Build history of the part. All positions in model axes, mm. A direction names the side the tool comes from. Round coordinates to 2 decimals unless told otherwise and drop trailing zeros. Order: outer loops, then holes, each group sorted by start corner. A loop starts at its lowest first (then second) coordinate and runs counter-clockwise, first axis right, second up. Notation, with made-up numbers: (29, 74.5) -> (64, 74.5) arc R30 cw to (64, 105.5) -> close; hole circle Ø10 at (84, 53.5). An arc over 180 degrees is marked (long way). Answer as a JSON object with one key per item and string values.
from build123d import *

# Parameters (mm, degrees)
BOSS_EXTRUDE1_DEPTH   = 3.175
BOSS_EXTRUDE2_DEPTH   = 3.175
F_4_CLEARANCE_HOLE1_D = 2.9464


with BuildPart() as part:
    # Sketch1 → Boss-Extrude1 (new body)
    with BuildSketch(Plane(origin=(0, 0, -14.15699402), x_dir=(-1, 0, 0), z_dir=(0, 0, -1))):
        with BuildLine():
            Line((-49.172312317, -34.502108483), (-53.141062317, -27.628031841))
            ThreePointArc((-53.141062317, -27.628031841), (-55.063803638, -24.012221257), (-56.72992661, -20.271224785))
            ThreePointArc((-56.72992661, -20.271224785), (-54.976138042, -16.13776671), (-50.842679967, -17.891555277))
            ThreePointArc((-50.842679967, -17.891555277), (-49.356678398, -21.228119699), (-47.641801003, -24.453031841))
            Line((-47.641801003, -24.453031841), (-43.673051003, -31.327108483))
            ThreePointArc((-43.673051003, -31.327108483), (-16.68272836, -52.037511462), (17.046778195, -47.596937682))
            Line((17.046778195, -47.596937682), (23.920854837, -43.628187682))
            Line((23.920854837, -43.628187682), (30.79493148, -39.659437682))
            ThreePointArc((30.79493148, -39.659437682), (51.505334458, -12.669115038), (47.064760678, 21.060391517))
            Line((47.064760678, 21.060391517), (43.096010678, 27.934468159))
            ThreePointArc((43.096010678, 27.934468159), (41.160593535, 31.032051618), (39.01404477, 33.987248938))
            ThreePointArc((39.01404477, 33.987248938), (39.561948355, 38.44382292), (44.018522337, 37.895919335))
            ThreePointArc((44.018522337, 37.895919335), (46.425258832, 34.58251628), (48.595271992, 31.109468159))
            Line((48.595271992, 31.109468159), (52.564021992, 24.235391517))
            ThreePointArc((52.564021992, 24.235391517), (57.638963455, -14.312615975), (33.96993148, -45.158698996))
            Line((33.96993148, -45.158698996), (27.095854837, -49.127448996))
            Line((27.095854837, -49.127448996), (20.221778195, -53.096198996))
            ThreePointArc((20.221778195, -53.096198996), (-18.326229296, -58.171140459), (-49.172312317, -34.502108483))
        make_face()
    extrude(amount=BOSS_EXTRUDE1_DEPTH)

    # Sketch6 → Boss-Extrude2 (add)
    with BuildSketch(Plane.XY.offset(-14.15699402)):
        Polygon((78.577241059, -56.126600757), (56.126600757, -78.577241059), (27.345741417, -49.796381719), (49.796381719, -27.345741417), align=None)
        with BuildLine():
            Line((62.053569797, -46.248319024), (64.873370219, -49.068119446))
            ThreePointArc((64.873370219, -49.068119446), (64.873370219, -64.873370219), (49.068119446, -64.873370219))
            Line((49.068119446, -64.873370219), (46.248319024, -62.053569797))
            ThreePointArc((46.248319024, -62.053569797), (46.248319024, -46.248319024), (62.053569797, -46.248319024))
        make_face(mode=Mode.SUBTRACT)
        with BuildLine():
            Line((55.946995634, -74.266718121), (53.127195212, -71.446917699))
            ThreePointArc((53.127195212, -71.446917699), (53.127195212, -69.399419304), (55.174693608, -69.399419304))
            Line((55.174693608, -69.399419304), (57.99449403, -72.219219726))
            ThreePointArc((57.99449403, -72.219219726), (57.99449403, -74.266718121), (55.946995634, -74.266718121))
        make_face(mode=Mode.SUBTRACT)
        with BuildLine():
            Line((38.902469516, -53.127195212), (41.722269938, -55.946995634))
            ThreePointArc((41.722269938, -55.946995634), (41.722269938, -57.99449403), (39.674771543, -57.99449403))
            Line((39.674771543, -57.99449403), (36.854971121, -55.174693608))
            ThreePointArc((36.854971121, -55.174693608), (36.854971121, -53.127195212), (38.902469516, -53.127195212))
        make_face(mode=Mode.SUBTRACT)
        with BuildLine():
            Line((55.174693608, -36.854971121), (57.99449403, -39.674771543))
            ThreePointArc((57.99449403, -39.674771543), (57.99449403, -41.722269938), (55.946995634, -41.722269938))
            Line((55.946995634, -41.722269938), (53.127195212, -38.902469516))
            ThreePointArc((53.127195212, -38.902469516), (53.127195212, -36.854971121), (55.174693608, -36.854971121))
        make_face(mode=Mode.SUBTRACT)
        with BuildLine():
            Line((71.446917699, -53.127195212), (74.266718121, -55.946995634))
            ThreePointArc((74.266718121, -55.946995634), (74.266718121, -57.99449403), (72.219219726, -57.99449403))
            Line((72.219219726, -57.99449403), (69.399419304, -55.174693608))
            ThreePointArc((69.399419304, -55.174693608), (69.399419304, -53.127195212), (71.446917699, -53.127195212))
        make_face(mode=Mode.SUBTRACT)
    extrude(amount=-BOSS_EXTRUDE2_DEPTH)

    # #4 Clearance Hole1 (through all)
    with Locations(Plane(origin=(0, 0, -17.33199402), x_dir=(-1, 0, 0), z_dir=(0, 0, -1))):
        with Locations((-53.56643166, -20.541270527), (-47.21643166, -31.539793155), (42.670641335, 35.021229473), (49.020641335, 24.022706845)):
            Hole(F_4_CLEARANCE_HOLE1_D / 2)


solid = part.part
1) Which spindle directions (+Z, -Z, +X, -X, +Y, -Y) get a long thin tool onto all of the face, cutting with end or side? Do faces 1 (the face through (65.11, -42.66, -15.72)), 2 (the face through (-50.55, 27.72, -15.72)), 3 (the face through (49.38, -21.18, -15.72)), 4 (the face through (-57.78, -13.77, -15.72)), 5 (the face through (47.678, -63.483, -15.722)). Say none if no direction does.
Checked values:
{"face 1": "+Z, -Z, +X", "face 2": "+Z, -Z, -X, +Y", "face 3": "+Z, -Z, +Y", "face 4": "+Z, -Z, -X", "face 5": "+Z, -Z"}
2) Flat gauge pin, fed straight in: pin 1 Ø1 at (y, z) = (6.5, -15) entering from -X. Where does the tip first touch, or does it go through?
Checked values:
{"pin 1": "stops at x = -58.86"}
3) Probe L1, parallel to X at y = -41.5, z = -16.85; L2, parallel to X at y = -72, z = -16.15; L3, parallel to X at y = -42.5, z = -14.9. List the from-to ranges inside material, lowest first. Write a range as from..to.
Checked values:
{"L1": "x = -39.45..-27.61, 35.61..55.72, 58.18..63.95", "L2": "x = 49.55..53.68, 57.78..62.7", "L3": "x = -38.1..-25.87, 34.51..64.95"}
4) Pull direction X, two halves, no side cores. Call faces 6 (the face through (5, -54, -14.157)), 7 (the face through (52.4, -21.44, -15.72)), 8 (the face through (-45.11, 24.45, -15.72)), 9 (the face through (-46.393, 34.63, -15.722)): pulls with the +X half, pulls with the -X half, needs draft (parallel to the pull), parting line crosses it, or undercut.
Checked values:
{"face 6": "needs draft", "face 7": "undercut", "face 8": "pulls with the +X half", "face 9": "pulls with the -X half"}
5) Cut at A-A, the plane y = 17.5. Give the cut face in (x, z), plus the area to 3 significant figures.
Checked values:
{"outline": "(-55.82, -17.33) -> (-48.91, -17.33) -> (-48.91, -14.16) -> (-55.82, -14.16) -> close", "area": "21.9 mm²"}
6) Cut at B-B, the plane z = -16.85. Count the separate pieces of the cut face and the enclosed holes in it, plus the area to 3 significant figures.
Checked values:
{"separate pieces": "1", "enclosed holes": "9", "area": "1,820 mm²"}
7) Cut at C-C, the plane x = 19.5. Give the cut face in (y, z).
Checked values:
{"outline": "(-57.84, -17.33) -> (-51.18, -17.33) -> (-51.18, -14.16) -> (-57.84, -14.16) -> close"}
